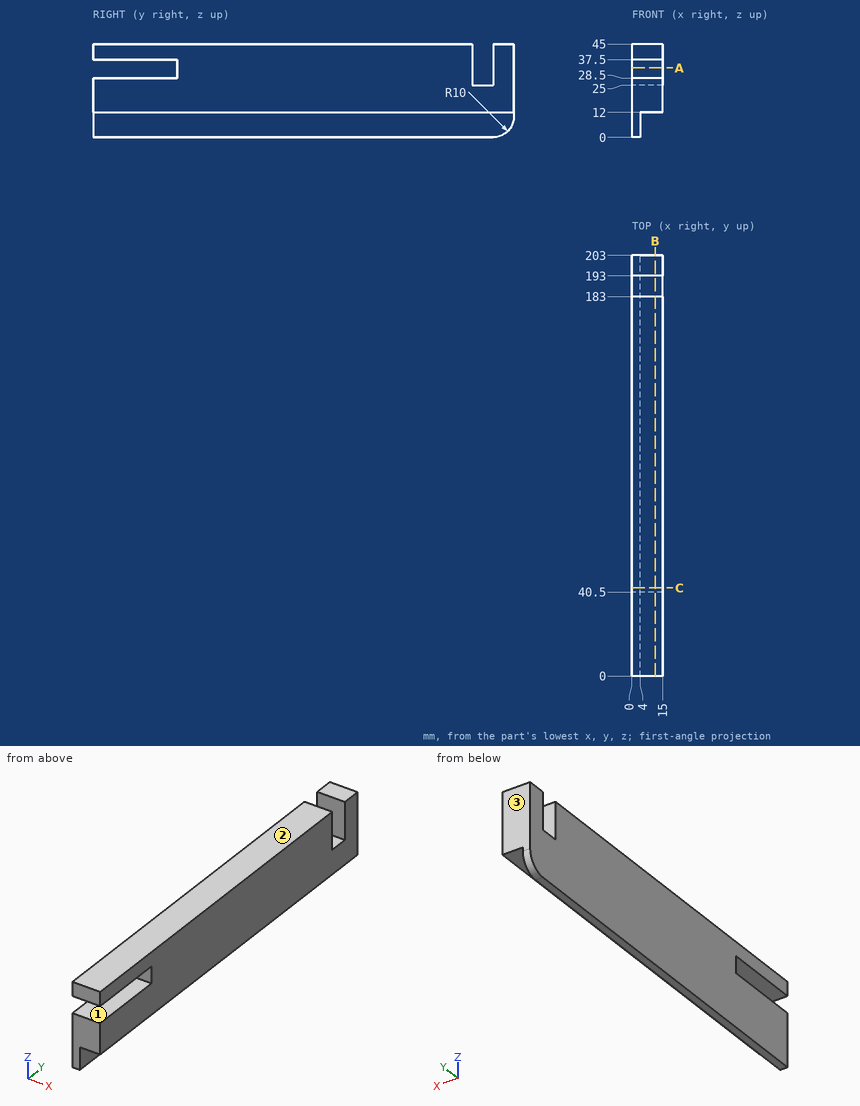
Input: dimensioned drawing with shaded views. Units: mm. Origin: part minimum x, y, z. Round coordinates to 2 decimals unless told otherwise and drop trailing zeros. Write each loop counter-clockwise with the first axis right and the second up, starting at its lowest first coordinate (ties: lowest second). Pieces come first, ordered by that corner, then holes. Notation, with made-up numbers: (35, 29) -> (83, 29) arc R17 ccw to (83, 33) -> close; hole circle Ø10 at (50.5, -9). An arc over 180 degrees is marked (long way). Use CSV: the item, a comma, the result in double quotes. Start each with the question number.
Q1. Section A-A (z = 33.5). Return loops of the section in (x, y), plus the area to 3 significant figures.
Q2. First-contact query: pin 1 Ø8 at (x, y) = (4.5, 188) entering from +Z; pin 2 Ø7.5 at (x, y) = (10.5, 16.5) entering from -Z; pin 3 Ø4.5 at (x, z) = (9.5, 33) entering from -Y. Flat tips, straight axial feed; report the tip coordinate or a pass-through.
Q3. Pull-direction query (Z, two-part tool) for the marked faces 1, 2 and 3; classes: pulls with the +Z half, pulls with the -Z half, needs draft (parallel to the pull), parting line crosses it, or undercut.
Q4. Section B-B (x = 11.25). Return loops of the section in (y, z).
Q5. Section C-C (y = 42.5). Return loops of the section in (x, z).
Q6. Line query: L1, parallel to Y at x = 10.25, z = 30.5; L2, parallel to Z at x = 1.5, y = 13; L3, parallel to Y at x = 8.25, z = 38. Output: solid intervals per line, ascending.
Result sheet:
1,outline,"(0, 40.5) -> (15, 40.5) -> (15, 183) -> (0, 183) -> close; (0, 193) -> (15, 193) -> (15, 203) -> (0, 203) -> close"
1,area,"2,290 mm²"
2,pin 1,"z = 25"
2,pin 2,"z = 12"
2,pin 3,"y = 40.5"
3,face 1,"undercut"
3,face 2,"pulls with the +Z half"
3,face 3,"needs draft"
4,outline,"(0, 12) -> (203, 12) -> (203, 45) -> (193, 45) -> (193, 25) -> (183, 25) -> (183, 45) -> (0, 45) -> (0, 37.5) -> (40.5, 37.5) -> (40.5, 28.5) -> (0, 28.5) -> close"
5,outline,"(0, 0) -> (4, 0) -> (4, 12) -> (15, 12) -> (15, 45) -> (0, 45) -> close"
6,L1,"40.5 to 183, 193 to 203"
6,L2,"0 to 28.5, 37.5 to 45"
6,L3,"0 to 183, 193 to 203"
